The model under review builds one solid part; all positions refer to its coordinate system, in mm. Face numbers are marked on the shaded views. A direction names the side the tool comes from. Round coordinates to 2 decimals unless told otherwise and drop trailing zeros. Write each loop counter-clockwise with the first axis right and the second up, starting at its lowest first coordinate (ties: lowest second). Pieces come first, ordered by that corner, then holes. Notation, with made-up numbers: (-11, -33) - (-5, -33) arc R19 ccw to (-5, -12) - close; hole circle Ø4 at (-33.5, 37). An arc over 180 degrees is marked (long way). Return JSON: item names as keys, results as strings.
from build123d import *

# Parameters (mm, degrees)
BOSS_EXTRUDE1_DEPTH  = 36.0172
SKETCH7_R            = 31.2928
BOSS_EXTRUDE4_DEPTH  = 36.0172
CUT_EXTRUDE2_START   = -6.35
CUT_EXTRUDE2_DEPTH   = 6.35
CUT_EXTRUDE3_DEPTH   = 10.795
SKETCH10_R           = 2.8067
BOSS_EXTRUDE5_DEPTH  = 5.4864
SKETCH11_R           = 20.6248
BOSS_EXTRUDE6_DEPTH  = 1.9558
SKETCH12_R           = 14.3637
BOSS_EXTRUDE7_DEPTH  = 32.3088
BOSS_EXTRUDE9_DEPTH  = 10.6934
SKETCH14_R           = 2.3495
CUT_EXTRUDE4_DEPTH   = 2.54
SKETCH15_W           = 27.051
SKETCH15_H           = 2.54
BOSS_EXTRUDE10_DEPTH = 11.3538
SKETCH16_R           = 2.3495
CUT_EXTRUDE5_DEPTH   = 2.54
SKETCH17_R           = 3.7846
BOSS_EXTRUDE11_DEPTH = 2.3622
SKETCH18_R           = 3.7846
BOSS_EXTRUDE13_DEPTH = 2.3622


with BuildPart() as part:
    # Sketch1 → Boss-Extrude1 (new body)
    with BuildSketch(Plane.XY):
        with BuildLine():
            ThreePointArc((36.843812273, 2.145016468), (0, 36.9062), (-36.843812273, 2.145016468))
            Line((-36.843812273, 2.145016468), (36.843812273, 2.145016468))
        make_face()
        with BuildLine():
            Line((36.843812273, 2.145016468), (-36.843812273, 2.145016468))
            Line((-36.843812273, 2.145016468), (-36.843812273, -2.145016468))
            ThreePointArc((-36.843812273, -2.145016468), (-33.44326867, -15.608183082), (-25.30834218, -26.861783532))
            Line((-25.30834218, -26.861783532), (25.30834218, -26.861783532))
            ThreePointArc((25.30834218, -26.861783532), (33.882903776, -14.629300398), (36.9062, 0))
            ThreePointArc((36.9062, 0), (36.890599771, 1.072961774), (36.843812273, 2.145016468))
        make_face()
        with BuildLine():
            Line((36.9062, -26.861783532), (36.9062, 0))
            ThreePointArc((36.9062, 0), (33.882903776, -14.629300398), (25.30834218, -26.861783532))
            Line((25.30834218, -26.861783532), (36.9062, -26.861783532))
        make_face()
        with BuildLine():
            ThreePointArc((-25.30834218, -26.861783532), (-33.44326867, -15.608183082), (-36.843812273, -2.145016468))
            Line((-36.843812273, -2.145016468), (-36.843812273, -26.861783532))
            Line((-36.843812273, -26.861783532), (-25.30834218, -26.861783532))
        make_face()
    extrude(amount=BOSS_EXTRUDE1_DEPTH)

    # Sketch7 → Boss-Extrude4 (add)
    with BuildSketch(Plane.XY.offset(36.0172)):
        with Locations((0, -3.81)):
            Circle(SKETCH7_R)
    extrude(amount=-BOSS_EXTRUDE4_DEPTH)

    # Sketch6 → Cut-Extrude2 (cut)
    with BuildSketch(Plane(origin=(0, 0, 0), x_dir=(-1, 0, 0), z_dir=(0, 0, -1)).offset(CUT_EXTRUDE2_START)):
        with BuildLine():
            Line((21.162575643, -26.861783532), (-21.162575643, -26.861783532))
            ThreePointArc((-21.162575643, -26.861783532), (0, -35.1028), (21.162575643, -26.861783532))
        make_face()
    extrude(amount=CUT_EXTRUDE2_DEPTH, mode=Mode.SUBTRACT)

    # Sketch9 → Cut-Extrude3 (cut)
    with BuildSketch(Plane.XY.offset(36.0172)):
        with BuildLine():
            Line((-21.162575643, -26.861783532), (21.162575643, -26.861783532))
            ThreePointArc((21.162575643, -26.861783532), (0, -35.1028), (-21.162575643, -26.861783532))
        make_face()
    extrude(amount=-CUT_EXTRUDE3_DEPTH, mode=Mode.SUBTRACT)

    # Sketch10 → Boss-Extrude5 (add)
    with BuildSketch(Plane(origin=(0, 0, 0), x_dir=(-1, 0, 0), z_dir=(0, 0, -1))):
        with Locations(Location((0, -3.81, 0), (0, 0, 180))):
            Circle(SKETCH10_R)
    extrude(amount=BOSS_EXTRUDE5_DEPTH)

    # Sketch11 → Boss-Extrude6 (add)
    with BuildSketch(Plane.XY.offset(36.0172)):
        with Locations((0, -3.81)):
            Circle(SKETCH11_R)
    extrude(amount=BOSS_EXTRUDE6_DEPTH)

    # Sketch12 → Boss-Extrude7 (add)
    with BuildSketch(Plane.XY.offset(37.973)):
        with Locations((0, -3.81)):
            Circle(SKETCH12_R)
    extrude(amount=BOSS_EXTRUDE7_DEPTH)

    # Sketch13 → Boss-Extrude9 (add)
    with BuildSketch(Plane.XY.offset(36.0172)):
        with BuildLine():
            Line((-32.6136, -18.1737), (-14.800895154, -18.1737))
            ThreePointArc((-14.800895154, -18.1737), (-15.900839256, -16.945664657), (-16.899186174, -15.6337))
            Line((-16.899186174, -15.6337), (-32.6136, -15.6337))
            Line((-32.6136, -15.6337), (-32.6136, -18.1737))
        make_face()
        with BuildLine():
            ThreePointArc((-16.899186174, -15.6337), (-15.900839256, -16.945664657), (-14.800895154, -18.1737))
            Line((-14.800895154, -18.1737), (-7.9756, -18.1737))
            Line((-7.9756, -18.1737), (-7.9756, -15.755948365))
            ThreePointArc((-7.9756, -15.755948365), (-8.065898573, -15.695165455), (-8.155733934, -15.6337))
            Line((-8.155733934, -15.6337), (-16.899186174, -15.6337))
        make_face()
        with BuildLine():
            Line((7.9756, -18.1737), (14.800895154, -18.1737))
            ThreePointArc((14.800895154, -18.1737), (15.900839256, -16.945664657), (16.899186174, -15.6337))
            Line((16.899186174, -15.6337), (8.155733934, -15.6337))
            ThreePointArc((8.155733934, -15.6337), (8.065898573, -15.695165455), (7.9756, -15.755948365))
            Line((7.9756, -15.755948365), (7.9756, -18.1737))
        make_face()
        with BuildLine():
            Line((14.800895154, -18.1737), (32.6136, -18.1737))
            Line((32.6136, -18.1737), (32.6136, -15.6337))
            Line((32.6136, -15.6337), (16.899186174, -15.6337))
            ThreePointArc((16.899186174, -15.6337), (15.900839256, -16.945664657), (14.800895154, -18.1737))
        make_face()
    extrude(amount=BOSS_EXTRUDE9_DEPTH)

    # Sketch14 → Cut-Extrude4 (cut)
    with BuildSketch(Plane(origin=(0, -15.6337, 0), x_dir=(1, 0, 0), z_dir=(0, 1, 0))):
        with Locations(Location((-24.2062, -40.8432, 0), (0, 0, 270))):
            Circle(SKETCH14_R)
        with Locations(Location((24.2062, -40.8432, 0), (0, 0, 270))):
            Circle(SKETCH14_R)
    extrude(amount=-CUT_EXTRUDE4_DEPTH, mode=Mode.SUBTRACT)

    # Sketch15 → Boss-Extrude10 (add)
    with BuildSketch(Plane(origin=(0, 0, 0), x_dir=(-1, 0, 0), z_dir=(0, 0, -1))):
        with Locations((-6.1595, -17.018)):
            Rectangle(SKETCH15_W, SKETCH15_H)
    extrude(amount=BOSS_EXTRUDE10_DEPTH)

    # Sketch16 → Cut-Extrude5 (cut)
    with BuildSketch(Plane(origin=(0, -15.748, 0), x_dir=(1, 0, 0), z_dir=(0, 1, 0))):
        with Locations(Location((5.698514736, 4.699, 0), (0, 0, 180))):
            Circle(SKETCH16_R)
    extrude(amount=-CUT_EXTRUDE5_DEPTH, mode=Mode.SUBTRACT)

    # Sketch17 → Boss-Extrude11 (add)
    with BuildSketch(Plane.XZ.offset(18.288)):
        with BuildLine():
            Line((0.072414736, -4.699), (0, 0))
            Line((0, 0), (11.324614736, 0))
            Line((11.324614736, 0), (11.324614736, -4.699))
            ThreePointArc((11.324614736, -4.699), (5.698514736, -10.3251), (0.072414736, -4.699))
        make_face()
        with Locations((5.698514736, -4.699)):
            Circle(SKETCH17_R, mode=Mode.SUBTRACT)
    extrude(amount=BOSS_EXTRUDE11_DEPTH)

    # Sketch18 → Boss-Extrude13 (add)
    # profile 1 of 2: a face of its own
    with BuildSketch(Plane.XZ.offset(18.1737)):
        with BuildLine():
            Line((-18.5801, 40.8432), (-18.5801, 36.0172))
            Line((-18.5801, 36.0172), (-29.8323, 36.0172))
            Line((-29.8323, 36.0172), (-29.8323, 40.8432))
            ThreePointArc((-29.8323, 40.8432), (-24.2062, 46.4693), (-18.5801, 40.8432))
        make_face()
        with Locations((-24.2062, 40.8432)):
            Circle(SKETCH18_R, mode=Mode.SUBTRACT)
    # profile 2 of 2: a face of its own
    with BuildSketch(Plane.XZ.offset(18.1737)):
        with BuildLine():
            Line((29.8323, 36.0172), (29.8323, 40.8432))
            ThreePointArc((29.8323, 40.8432), (24.2062, 46.4693), (18.5801, 40.8432))
            Line((18.5801, 40.8432), (18.5801, 36.0172))
            Line((18.5801, 36.0172), (29.8323, 36.0172))
        make_face()
        with Locations((24.2062, 40.8432)):
            Circle(SKETCH18_R, mode=Mode.SUBTRACT)
    extrude(amount=BOSS_EXTRUDE13_DEPTH)


solid = part.part
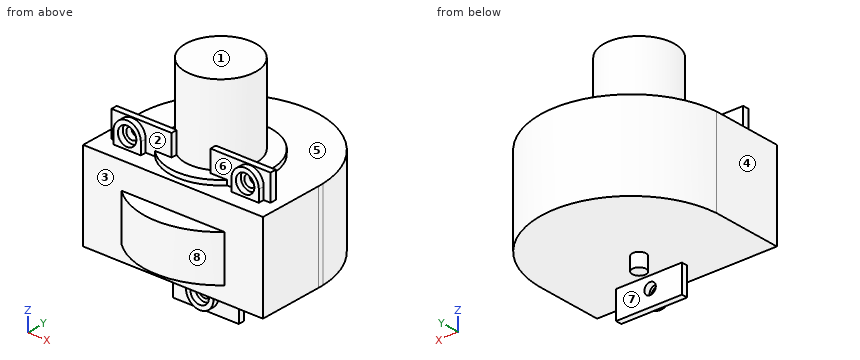
(1) Add section A-A (y = -3.81). Write out the cut boundary in (x, z).
Filled in:
{"outline": "(-36.84, 0) - (-2.81, 0) - (-2.81, -5.49) - (2.81, -5.49) - (2.81, 0) - (36.91, 0) - (36.91, 36.02) - (20.62, 36.02) - (20.62, 37.97) - (14.36, 37.97) - (14.36, 70.28) - (-14.36, 70.28) - (-14.36, 37.97) - (-20.62, 37.97) - (-20.62, 36.02) - (-36.84, 36.02) - close"}
(2) Clearance check with flat-ended pins moving along their axes: pin 1 Ø8 at (x, z) = (15, 43.5) entering from +Y; pin 2 Ø1.9 at (y, z) = (-19.5, 38) entering from +X; pin 3 Ø4 at (x, z) = (6.5, 19.5) entering from -Y. State where each tip first meets the part, or that it passes through.
Filled in:
{"pin 1": "stops at y = 5.43", "pin 2": "stops at x = 29.83", "pin 3": "stops at y = -34.78"}
(3) Add section D-D (x = -10). Write out the cut boundary in (y, z).
Filled in:
{"outline": "(-33.46, 6.35) - (-26.86, 6.35) - (-26.86, 0) - (35.53, 0) - (35.53, 36.02) - (14.23, 36.02) - (14.23, 37.97) - (6.5, 37.97) - (6.5, 70.28) - (-14.12, 70.28) - (-14.12, 37.97) - (-15.63, 37.97) - (-15.63, 46.71) - (-18.17, 46.71) - (-18.17, 37.97) - (-21.85, 37.97) - (-21.85, 36.02) - (-26.86, 36.02) - (-26.86, 25.22) - (-33.46, 25.22) - close"}
(4) Mouldability with a two-part tool opening along X and no side actions: class the marked faces 6, 7 and 8 as released by +X, released by -X, zero draft, split by the parting line, or undercut.
Filled in:
{"face 6": "undercut", "face 7": "zero draft", "face 8": "split by the parting line"}
(5) Wall thickness on line 1 (Z direction, x = -8.5, y = 1); line 2 (Z direction, x = -13.5, y = 13); line 3 (Y direction, x = 34, z = 12): over which ranges is each line inside the solid? List them lowest first.
Filled in:
{"line 1": "z = 0 to 70.28", "line 2": "z = 0 to 36.02", "line 3": "y = -26.86 to 14.36"}
(6) Add section B-B (z = 42). Give the number of separate pieces and of enclosed holes in the cut face, plus the area to 4 significant figures.
Filled in:
{"separate pieces": "3", "enclosed holes": "0", "area": "770.5 mm2"}
(7) Add section C-C (z = 52). Write out the cut boundary in (x, y).
Filled in:
{"outline": "circle Ø28.73 at (0, -3.81)"}
(8) For the marked faces 1, 2, 3, 4 and 5, list the 3-axis set-ups (+Z, -Z, +X, -X, +Y, -Y) from which the entire face can be reached by the end or side of a thin tool; tool diameter is ignored.
Filled in:
{"face 1": "+Z, +X, -X, +Y, -Y", "face 2": "+Z, -Y", "face 3": "-Y", "face 4": "+Z, -Z, -X, +Y, -Y", "face 5": "+Z"}
